from build123d import *

# Parameters (mm, degrees)
BOSS_EXTRUDE1_DEPTH = 38.1
SKETCH2_R           = 5
SKETCH2_R_2         = 3.175
CUT_EXTRUDE1_DEPTH  = 319.018514003
SKETCH3_W           = 293.188888759
SKETCH3_H           = 137.971241769
CUT_EXTRUDE2_DEPTH  = 319.018514003
SKETCH4_R           = 7
CUT_EXTRUDE3_DEPTH  = 3.175
SKETCH5_W           = 61.216236185
SKETCH5_H           = 51.695253477
CUT_EXTRUDE4_DEPTH  = 65.391872686


with BuildPart() as part:
    # Sketch1 → Boss-Extrude1 (new body)
    with BuildSketch(Plane.XY):
        with BuildLine():
            add(Edge.make_bspline(
                [(0.000560351, 0.000130087), (0.810633127, 7.359196055), (8.649092025, 17.856605174), (26.286719818, 29.975176328), (52.111128271, 42.069215275), (89.597618475, 49.290763054), (131.400792109, 47.884831915), (173.256699242, 40.041104278), (217.961060472, 29.612974894), (256.952064401, 19.528920948), (290.35983767, 8.71099439), (301.273197721, 4.382828139), (314.816918223, -0.516206742), (309.846313895, 0.000130087)],
                knots=[0, 0, 0, 0, 0.060863618, 0.113688265, 0.188608742, 0.312908923, 0.448482434, 0.557612135, 0.691544113, 0.852438279, 0.92975597, 0.976058229, 1, 1, 1, 1], degree=3))
            add(Edge.make_bspline(
                [(309.846313895, 0.000130087), (303.956832565, 1.47095521), (293.989507544, 2.093987313), (276.26402299, 4.514356704), (260.846344817, 5.427413394), (235.858814759, 7.870306192), (205.101424636, 8.838080282), (157.718638092, 9.030650149), (110.497331172, 6.181495223), (66.506197185, -0.586669107), (36.454672816, -6.098499901), (15.316603331, -6.189065841), (1.230714189, -6.924076091), (0.000560351, 0.000130087)],
                knots=[0, 0, 0, 0, 0.057787081, 0.095274891, 0.171021118, 0.205339302, 0.335319146, 0.464904334, 0.658702312, 0.785511947, 0.893517288, 0.94309214, 1, 1, 1, 1], degree=3))
        make_face()
    boss_extrude1 = extrude(amount=BOSS_EXTRUDE1_DEPTH)

    # Sketch2 → Cut-Extrude1 (cut, through all)
    with BuildSketch(Plane.XY.offset(38.1)):
        with Locations((20.32, 10.16)):
            Circle(SKETCH2_R)
        with Locations((227.296313895, 19.050130087)):
            Circle(SKETCH2_R_2)
    cut_extrude1 = extrude(amount=-CUT_EXTRUDE1_DEPTH, mode=Mode.SUBTRACT)

    # Sketch3 → Cut-Extrude2 (cut, through all)
    with BuildSketch(Plane.XY.offset(38.1)):
        with Locations((184.69444438, 2.732377951)):
            Rectangle(SKETCH3_W, SKETCH3_H)
    cut_extrude2 = extrude(amount=-CUT_EXTRUDE2_DEPTH, mode=Mode.SUBTRACT)

    # Sketch4 → Cut-Extrude3 (cut)
    with BuildSketch(Plane(origin=(0, 0, 0), x_dir=(-1, 0, 0), z_dir=(0, 0, -1))):
        with Locations((-20.32, 10.16)):
            Circle(SKETCH4_R)
    cut_extrude3 = extrude(amount=-CUT_EXTRUDE3_DEPTH, mode=Mode.SUBTRACT)

    # Mirror1: Boss-Extrude1, Cut-Extrude1, Cut-Extrude2, Cut-Extrude3 across plane
    add(boss_extrude1.mirror(Plane(origin=(153.387816973, 8.333381989, 0), x_dir=(1, 0, 0), z_dir=(0, 0, -1))))
    add(cut_extrude1.mirror(Plane(origin=(153.387816973, 8.333381989, 0), x_dir=(1, 0, 0), z_dir=(0, 0, -1))), mode=Mode.SUBTRACT)
    add(cut_extrude2.mirror(Plane(origin=(153.387816973, 8.333381989, 0), x_dir=(1, 0, 0), z_dir=(0, 0, -1))), mode=Mode.SUBTRACT)
    add(cut_extrude3.mirror(Plane(origin=(153.387816973, 8.333381989, 0), x_dir=(1, 0, 0), z_dir=(0, 0, -1))), mode=Mode.SUBTRACT)

    # Sketch5 → Cut-Extrude4 (cut, through all)
    with BuildSketch(Plane(origin=(38.1, 0, 0), x_dir=(0, 0, -1), z_dir=(1, 0, 0))):
        with Locations((-30.608118093, 9.410506282)):
            Rectangle(SKETCH5_W, SKETCH5_H)
    extrude(amount=-CUT_EXTRUDE4_DEPTH, mode=Mode.SUBTRACT)


solid = part.part
Here's how the part is built. I have some questions about the finished solid (model axes, mm). A direction names the side the tool comes from. Coordinates: 2 decimals unless noted, no trailing zeros.
1. For P1, Ø12, axis at x = 29, z = -25.5, coming from the -Y side; P2, Ø8, axis at y = 16.5, z = -9, coming from the -X side; P3, Ø2, axis at y = 8, z = -23, coming from the -X side; P4, Ø8, axis at x = 20.32, y = 10.16, coming from the -Z side, each with a flat end and sliding along its axis, tell me the tip position at first contact or that it passes through.
2. For faces 3 (the flat face through (28, 9, 0)), 4 (the flat face through (16, 7, -3.175)), which set-ups out of +Z, -Z, +X, -X, +Y, -Y let a thin tool reach every point of the face, with its end or its side?
3. If we mould it in two halves opening along Y, with no side actions, what happens to faces 1 (the flat face through (24, 5, -38.1)), 2 (the cylindrical face through (27.313, 10.468, -1.565))? For each: pulls with the +Y half, pulls with the -Y half, needs draft (parallel to the pull), parting line crosses it, or undercut.
4. I need wall thicknesses on L1, parallel to X at y = 10, z = -1; L2, parallel to X at y = 7, z = -5; L3, parallel to Y at x = 20.32, z = -1.65. Which ranges of each line are inside material? Lowest first, please.
Taken from the geometry:
1. P1: stops at y = -6.14
1. P2: stops at x = 5.26
1. P3: stops at x = 1.93
1. P4: passes through
2. face 3: +Z, +X, -X, +Y, -Y
2. face 4: +Z
3. face 1: needs draft
3. face 2: undercut
4. L1: x = 3.53 to 13.32, 27.32 to 38.1
4. L2: x = 1.93 to 16.45, 24.19 to 38.1
4. L3: y = -6.21 to 3.16, 17.16 to 25.66
